Study the drawing (mm; zero at the part's minimum x, y, z) and answer. Round coordinates to 2 decimals unless told otherwise and drop trailing zeros. Loops run counter-clockwise (first coordinate to the right, second up) from the corner with the lowest first, then second, coordinate; pieces in that order, holes last. Notation, with made-up numbers: (43.25, -29.5) - (78.25, -29.5) arc R31 cw to (78.25, 9.5) - close; hole circle Ø2 at (-24, 82). An arc over 180 degrees is marked (long way). Use CSV: the item, a comma, the result in double quotes. Start each with the question number.
1. Determine the mould class of the marked faces 1, 2, 3 and 4 for opening direction X: +X half, -X half, draft (parallel to the pull), parting line (faces both ways), or undercut.
2. Find section C-C (z = 36.75). Give the vertices of the cut face in (x, y).
3. Consider line 1 along X through (y, z) = (21.5, 14.5); line 2 along Y through (x, z) = (32.5, 3); line 3 along Y through (x, z) = (57.5, 13.25) (1 decimal). Determine where each line is inside the solid, lowest interval first.
4. Find section B-B (y = 14.5). Give the vertices of the cut face in (x, z).
5. Given pin 1 Ø8 at (y, z) = (14.5, 13.25) entering from +X; pin 2 Ø7 at (y, z) = (14.5, 36.75) entering from -X, each flat-ended and moving along its own axis, determine where each tip first touches the part or whether it passes through.
6. Find section A-A (y = 27). Give the vertices of the cut face in (x, z).
7. Find section D-D (z = 5). Give the vertices of the cut face in (x, y).
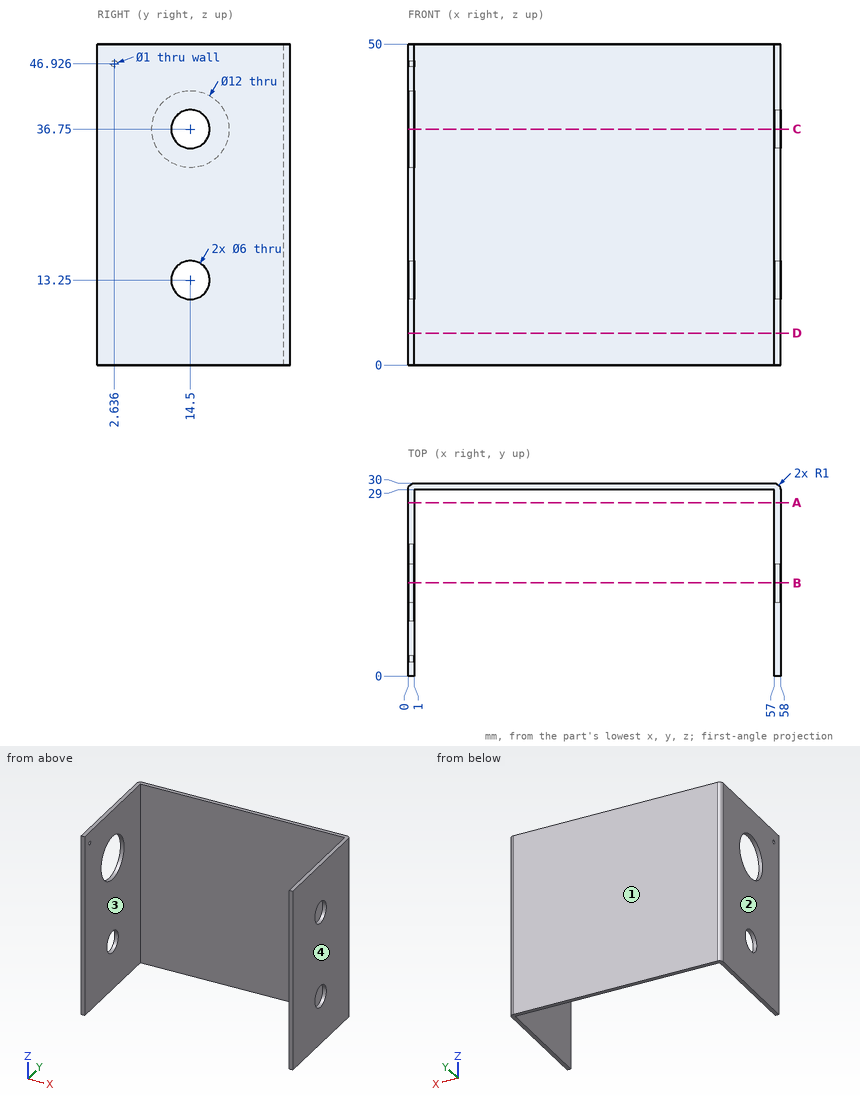
Filled sheet:
1,face 1,"draft"
1,face 2,"-X half"
1,face 3,"undercut"
1,face 4,"+X half"
2,outline,"(0, 0) - (1, 0) - (1, 8.5) - (0, 8.5) - close; (0, 20.5) - (1, 20.5) - (1, 29) - (57, 29) - (57, 17.5) - (58, 17.5) - (58, 29) arc R1 ccw to (57, 30) - (1, 30) arc R1 ccw to (0, 29) - close; (57, 0) - (58, 0) - (58, 11.5) - (57, 11.5) - close"
3,line 1,"x = 0 to 1, 57 to 58"
3,line 2,"y = 29 to 30"
3,line 3,"y = 0 to 11.5, 17.5 to 29.9"
4,outline,"(0, 0) - (1, 0) - (1, 10.25) - (0, 10.25) - close; (0, 16.25) - (1, 16.25) - (1, 30.75) - (0, 30.75) - close; (0, 42.75) - (1, 42.75) - (1, 50) - (0, 50) - close; (57, 0) - (58, 0) - (58, 10.25) - (57, 10.25) - close; (57, 16.25) - (58, 16.25) - (58, 33.75) - (57, 33.75) - close; (57, 39.75) - (58, 39.75) - (58, 50) - (57, 50) - close"
5,pin 1,"stops at x = 58"
5,pin 2,"stops at x = 57"
6,outline,"(0, 0) - (1, 0) - (1, 50) - (0, 50) - close; (57, 0) - (58, 0) - (58, 50) - (57, 50) - close"
7,outline,"(0, 0) - (1, 0) - (1, 29) - (57, 29) - (57, 0) - (58, 0) - (58, 29) arc R1 ccw to (57, 30) - (1, 30) arc R1 ccw to (0, 29) - close"
